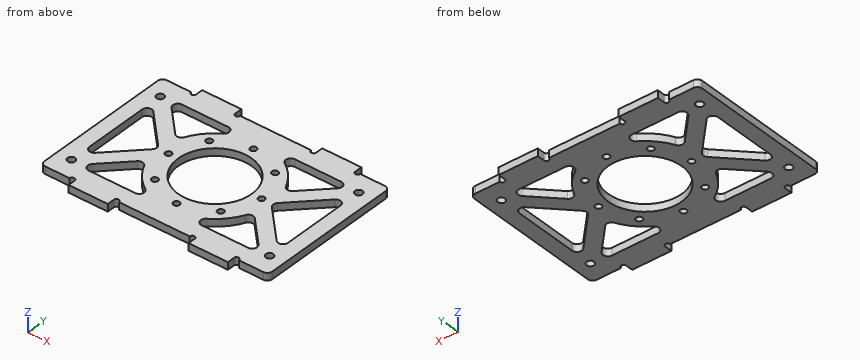
```python
from build123d import *

# Parameters (mm, degrees)
SKETCH_1_W               = 93
SKETCH_1_H               = 60
EXTRUDE_1_DEPTH          = 1.5
SKETCH_2_R               = 15
CUT_EXTRUDE_1_DEPTH      = 12
SKETCH_4_R               = 1.525
CUT_EXTRUDE_3_DEPTH      = 15
SKETCH_5_R               = 1.275
CUT_EXTRUDE_4_DEPTH      = 15
CUT_EXTRUDE_7_DEPTH      = 10
FILLET_3_R               = 2
FILLET_3_OF_MIRROR_3_R   = 2
FILLET_4_R               = 2
SKETCH_10_W              = 16
SKETCH_10_H              = 6
EXTRUDE_2_DEPTH          = 3
MIRROR_5_COPY_1_SKETCH_W = 16
MIRROR_5_COPY_1_SKETCH_H = 6
MIRROR_5_COPY_1_DEPTH    = 3
SKETCH_11_R              = 1.025
CUT_EXTRUDE_8_DEPTH      = 3


with BuildPart() as part:
    # 草图1 → 凸台-拉伸1 (new body, symmetric)
    with BuildSketch(Plane.XY):
        Rectangle(SKETCH_1_W, SKETCH_1_H)
    extrude(amount=EXTRUDE_1_DEPTH, both=True)

    # 草图2 → 切除-拉伸1 (cut, symmetric)
    with BuildSketch(Plane.XY.offset(1.5)):
        Circle(SKETCH_2_R)
    extrude(amount=CUT_EXTRUDE_1_DEPTH, both=True, mode=Mode.SUBTRACT)

    # 草图4 → 切除-拉伸3 (cut, symmetric)
    with BuildSketch(Plane.XY.offset(1.5)):
        with Locations((40.5, -22)):
            Circle(SKETCH_4_R)
        with Locations((40.5, 22)):
            Circle(SKETCH_4_R)
        with Locations((-40.5, -22)):
            Circle(SKETCH_4_R)
        with Locations((-40.5, 22)):
            Circle(SKETCH_4_R)
    extrude(amount=CUT_EXTRUDE_3_DEPTH, both=True, mode=Mode.SUBTRACT)

    # 草图5 → 切除-拉伸4 (cut, symmetric)
    with BuildSketch(Plane.XY.offset(1.5)):
        with Locations((0, 19)):
            Circle(SKETCH_5_R)
        with Locations((13.435028843, 13.435028843)):
            Circle(SKETCH_5_R)
        with Locations((19, 0)):
            Circle(SKETCH_5_R)
        with Locations((13.435028843, -13.435028843)):
            Circle(SKETCH_5_R)
        with Locations((0, -19)):
            Circle(SKETCH_5_R)
        with Locations((-13.435028843, -13.435028843)):
            Circle(SKETCH_5_R)
        with Locations((-19, 0)):
            Circle(SKETCH_5_R)
        with Locations((-13.435028843, 13.435028843)):
            Circle(SKETCH_5_R)
    extrude(amount=CUT_EXTRUDE_4_DEPTH, both=True, mode=Mode.SUBTRACT)

    # 草图9 → 切除-拉伸7 (cut)
    with BuildSketch(Plane.XY.offset(1.5)):
        Polygon((40.5, 17.906976744), (23, 0), (40.5, -17.906976744), align=None)
        with BuildLine():
            Line((37.282566796, 23), (21.843403436, 7.201786329))
            ThreePointArc((21.843403436, 7.201786329), (13.478852222, 18.636537843), (0, 23))
            Line((0, 23), (37.282566796, 23))
        make_face()
        with BuildLine():
            Line((37.282566796, -23), (0, -23))
            ThreePointArc((0, -23), (13.478852222, -18.636537843), (21.843403436, -7.201786329))
            Line((21.843403436, -7.201786329), (37.282566796, -23))
        make_face()
    cut_extrude_7 = extrude(amount=-CUT_EXTRUDE_7_DEPTH, mode=Mode.SUBTRACT)

    # 圆角3
    fillet_3_edges = [part.edges().sort_by_distance(p)[0] for p in [
        (0, -23, 0),
        (21.843403436, -7.201786329, 0),
        (37.282566796, -23, 0),
        (0, 23, 0),
        (37.282566796, 23, 0),
        (21.843403436, 7.201786329, 0),
        (40.5, 17.906976744, 0),
        (40.5, -17.906976744, 0),
        (23, 0, 0),
    ]]
    fillet(fillet_3_edges, radius=FILLET_3_R)

    # 镜向3: 切除-拉伸7 across plane
    add(cut_extrude_7.mirror(Plane(origin=(0, 0, 0), x_dir=(0, 0, 1), z_dir=(1, 0, 0))), mode=Mode.SUBTRACT)

    # 圆角3 of 镜向3
    fillet_3_of_mirror_3_edges = [part.edges().sort_by_distance(p)[0] for p in [
        (0, -23, 0),
        (-21.843403436, -7.201786329, 0),
        (-37.282566796, -23, 0),
        (0, 23, 0),
        (-37.282566796, 23, 0),
        (-21.843403436, 7.201786329, 0),
        (-40.5, 17.906976744, 0),
        (-40.5, -17.906976744, 0),
        (-23, 0, 0),
    ]]
    fillet(fillet_3_of_mirror_3_edges, radius=FILLET_3_OF_MIRROR_3_R)

    # 圆角4
    fillet_4_edges = [part.edges().sort_by_distance(p)[0] for p in [
        (46.5, -30, 0),
        (-46.5, -30, 0),
        (-46.5, 30, 0),
        (46.5, 30, 0),
    ]]
    fillet(fillet_4_edges, radius=FILLET_4_R)

    # 草图10 → 凸台-拉伸2 (add)
    with BuildSketch(Plane(origin=(0, 0, -1.5), x_dir=(-1, 0, 0), z_dir=(0, 0, -1))):
        with Locations((-24.5, 30)):
            Rectangle(SKETCH_10_W, SKETCH_10_H)
    extrude_2 = extrude(amount=-EXTRUDE_2_DEPTH)

    # 镜向4: 凸台-拉伸2 across plane
    add(extrude_2.mirror(Plane(origin=(0, 0, 0), x_dir=(0, 0, 1), z_dir=(1, 0, 0))))

    # 镜向5: 凸台-拉伸2 across plane
    add(extrude_2.mirror(Plane.ZX))

    # 镜向5 copy 1 sketch → 镜向5 copy 1 (add)
    with BuildSketch(Plane(origin=(0, 0, -1.5), x_dir=(1, 0, 0), z_dir=(0, 0, -1))):
        with Locations((-24.5, 30)):
            Rectangle(MIRROR_5_COPY_1_SKETCH_W, MIRROR_5_COPY_1_SKETCH_H)
    extrude(amount=-MIRROR_5_COPY_1_DEPTH)

    # 草图11 → 切除-拉伸8 (cut)
    with BuildSketch(Plane.XY.offset(1.5)):
        with Locations((33.525, 30)):
            Circle(SKETCH_11_R)
        with Locations((15.475, 30)):
            Circle(SKETCH_11_R)
        with Locations((-15.475, 30)):
            Circle(SKETCH_11_R)
        with Locations((-33.525, 30)):
            Circle(SKETCH_11_R)
        with Locations((-33.525, -30)):
            Circle(SKETCH_11_R)
        with Locations((-15.475, -30)):
            Circle(SKETCH_11_R)
        with Locations((15.475, -30)):
            Circle(SKETCH_11_R)
        with Locations((33.525, -30)):
            Circle(SKETCH_11_R)
    extrude(amount=-CUT_EXTRUDE_8_DEPTH, mode=Mode.SUBTRACT)


solid = part.part
```
Part model, mm, in its own coordinate system. Give positions to 0.01 mm unless a question says otherwise; leave off trailing zeros. Write each loop counter-clockwise with the first axis right and the second up, starting at its lowest first coordinate (ties: lowest second). Pieces come first, ordered by that corner, then holes. Notation, with made-up numbers: M 84.25,-19 L 140.25,-19 A8 ccw 140.25,-15 Z; hole C 36.5,-19.75 d8. An arc over 180 degrees is marked long. Use CSV: the item, a comma, the result in double quotes.
Item 1: Slice it at D-D on x = 0. Write the cut outline in (y, z) (3 decimals).
Taken from the geometry:
outline,"M -30,-1.5 L -20.275,-1.5 L -20.275,1.5 L -30,1.5 Z; M -17.725,-1.5 L -15,-1.5 L -15,1.5 L -17.725,1.5 Z; M 15,-1.5 L 17.725,-1.5 L 17.725,1.5 L 15,1.5 Z; M 20.275,-1.5 L 30,-1.5 L 30,1.5 L 20.275,1.5 Z"
Item 2: Slice it at A-A on y = 0. Write the cut outline in (x, z) (3 decimals).
Taken from the geometry:
outline,"M -46.5,-1.5 L -40.5,-1.5 L -40.5,1.5 L -46.5,1.5 Z; M -23.796,-1.5 L -20.275,-1.5 L -20.275,1.5 L -23.796,1.5 Z; M -17.725,-1.5 L -15,-1.5 L -15,1.5 L -17.725,1.5 Z; M 15,-1.5 L 17.725,-1.5 L 17.725,1.5 L 15,1.5 Z; M 20.275,-1.5 L 23.796,-1.5 L 23.796,1.5 L 20.275,1.5 Z; M 40.5,-1.5 L 46.5,-1.5 L 46.5,1.5 L 40.5,1.5 Z"
Item 3: Pin check, flat tips, straight feed: P1, Ø1, axis at x = -12.5, y = 5.5, coming from the -Z side; P2, Ø1.5, axis at y = 31.5, z = -0.5, coming from the -X side; P3, Ø3.5, axis at x = -13.44, y = -13.44, coming from the +Z side; P4, Ø0.9, axis at y = -31.5, z = -0.5, coming from the +X side. Stop position of each tip, or through.
Taken from the geometry:
P1,"passes through"
P2,"stops at x = -32.5"
P3,"stops at z = 1.5"
P4,"stops at x = 32.5"
Item 4: Slice it at C-C on y = 22. Write the cut outline in (x, z) (3 decimals), plus the area to 3 significant figures.
Taken from the geometry:
outline,"M -46.5,-1.5 L -42.025,-1.5 L -42.025,1.5 L -46.5,1.5 Z; M -38.975,-1.5 L -34.264,-1.5 L -34.264,1.5 L -38.975,1.5 Z; M -11.833,-1.5 L 11.833,-1.5 L 11.833,1.5 L -11.833,1.5 Z; M 34.264,-1.5 L 38.975,-1.5 L 38.975,1.5 L 34.264,1.5 Z; M 42.025,-1.5 L 46.5,-1.5 L 46.5,1.5 L 42.025,1.5 Z"
area,"126 mm²"
Item 5: Drill centre lines: probe 1 along X at (y, z) = (-7.5, 1.2); probe 2 along X at (y, z) = (-19.5, -1.1); probe 3 along Y at (x, z) = (-19, 0.1) (3 decimals). Where is each one in solid material? Low to high.
Taken from the geometry:
probe 1,"x = -46.5 to -40.5, -30.33 to -12.99, 12.99 to 30.33, 40.5 to 46.5"
probe 2,"x = -46.5 to -33.86, -12.24 to -1.17, 1.17 to 12.24, 33.86 to 46.5"
probe 3,"y = -33 to -23, -12.961 to -1.275, 1.275 to 12.961, 23 to 33"
Item 6: Slice it at B-B on x = 26. Write the cut outline in (y, z).
Taken from the geometry:
outline,"M -33,-1.5 L -23,-1.5 L -23,1.5 L -33,1.5 Z; M -11.46,-1.5 L -3.07,-1.5 L -3.07,1.5 L -11.46,1.5 Z; M 3.07,-1.5 L 11.46,-1.5 L 11.46,1.5 L 3.07,1.5 Z; M 23,-1.5 L 33,-1.5 L 33,1.5 L 23,1.5 Z"
